For this review, take the finished solid that the model builds, in its own axes (mm). A direction names the side the tool comes from. Give positions to 0.01 mm unless a question says otherwise; leave off trailing zeros. Write each loop counter-clockwise with the first axis right and the second up, starting at its lowest first coordinate (ties: lowest second). Pieces come first, ordered by that corner, then holes. Notation, with made-up numbers: M 87,-22.75 L 115,-22.75 A30 cw 115,11.25 Z; hole C 88.25,-39.5 d6. An arc over 180 degrees is marked long. One line per item, written item: value. Start each with the question number.
Item 1: Tool access review of faces 1 (the face through (-0.534, 4.065, -1.78)), 2 (the face through (-2.38, -10.74, 1.01)): name each direction out of +Z, -Z, +X, -X, +Y, -Y from which nothing blocks a thin tool from reaching the whole face with its end or side.
Item 2: Clearance check with flat-ended pins moving along their axes: pin 1 Ø10 at (x, y) = (7.5, 5.5) entering from -Z; pin 2 Ø2 at (x, z) = (-4.5, 0) entering from -Y; pin 3 Ø1.5 at (x, y) = (-4.5, -7.5) entering from -Z. State where each tip first meets the part, or that it passes through.
Item 3: Consider section A-A, the plane y = 0. Write out the cut boundary in (x, z).
Item 4: Consider section C-C, the plane z = -2.25. Write out the cut boundary in (x, y).
Item 5: To check wall thickness, follow probe 1 along Z at (x, y) = (4.75, 2.75); probe 2 along Z at (x, y) = (-5, 8.25); probe 3 along X at (y, z) = (-0.25, -2.4). State the ranges of each line that lie inside material, in increasing order.
```python
from build123d import *

# Parameters (mm, degrees)
F0_W   = 4.1
F0_H   = 0.4
F0_W_2 = 1.9
F0_H_2 = 2.8
F2_R   = 0.5


with BuildPart() as f1:
    # F0 (on Front) → F1 (revolve)
    with BuildSketch(Plane.XZ):
        Polygon((0, 2), (0, 0), (4.1, 0), (6, 0), (11, 0), (11, 2), align=None)
        with Locations((2.05, -0.2)):
            Rectangle(F0_W, F0_H)
        with Locations((5.05, -0.2)):
            Rectangle(F0_W_2, F0_H)
        with Locations((2.05, -1.8)):
            Rectangle(F0_W, F0_H_2)
    revolve(axis=Axis((0, 0, 1), (0, 0, 1)))

    # F2
    f2_edges = [f1.edges().sort_by_distance(p)[0] for p in [
        (-11, 0, 0),
        (-11, 0, 2),
    ]]
    fillet(f2_edges, radius=F2_R)


solid = f1.part
```
Model answer:
1. face 1: -Z
1. face 2: +Z, -Z
2. pin 1: stops at z = -0.4
2. pin 2: stops at y = -10.39
2. pin 3: stops at z = 0
3. outline: M -11,0.5 A0.5 ccw -10.5,0 L -6,0 L -6,-0.4 L -4.1,-0.4 L -4.1,-3.2 L 4.1,-3.2 L 4.1,-0.4 L 6,-0.4 L 6,0 L 10.5,0 A0.5 ccw 11,0.5 L 11,1.5 A0.5 ccw 10.5,2 L -10.5,2 A0.5 ccw -11,1.5 Z
4. outline: C 0,0 d8.2
5. probe 1: z = -0.4 to 2
5. probe 2: z = 0 to 2
5. probe 3: x = -4.09 to 4.09
